Design review of the part shown in the three views and the two pictorial views. Dimensions are in mm from the part's minimum x, y and z. Round coordinates to 2 decimals unless told otherwise and drop trailing zeros. Loops run counter-clockwise (first coordinate to the right, second up) from the corner with the lowest first, then second, coordinate; pieces in that order, holes last. Notation, with made-up numbers: M 13,-2.75 L 18,-2.75 A32 ccw 18,24.25 Z; hole C 21.25,73.5 d10. An arc over 180 degrees is marked long. Return JSON: item names as keys, results as strings. Group by question number.
Q1. Consider section A-A (x = 7.5). State the section outline as (y, z) points.
Q2. To check wall thickness, follow line 1 along Z through (x, y) = (42.5, 3); line 2 along X through (y, z) = (1.65, 14); line 3 along X through (y, z) = (0.7, 22). State the ranges of each line that lie inside material, in increasing order.
Q3. Consider section B-B (z = 15). State the section outline as (x, y) points, and give its area (3 significant figures).
Q4. Clearance check with a flat-ended pin moving along its axis: pin 1 Ø4.5 at (x, z) = (24.5, 12) entering from -Y. State where the tip first meets the part, or that it passes through.
Q5. Consider section C-C (x = 24). State the section outline as (y, z) points, and give its area (3 significant figures).
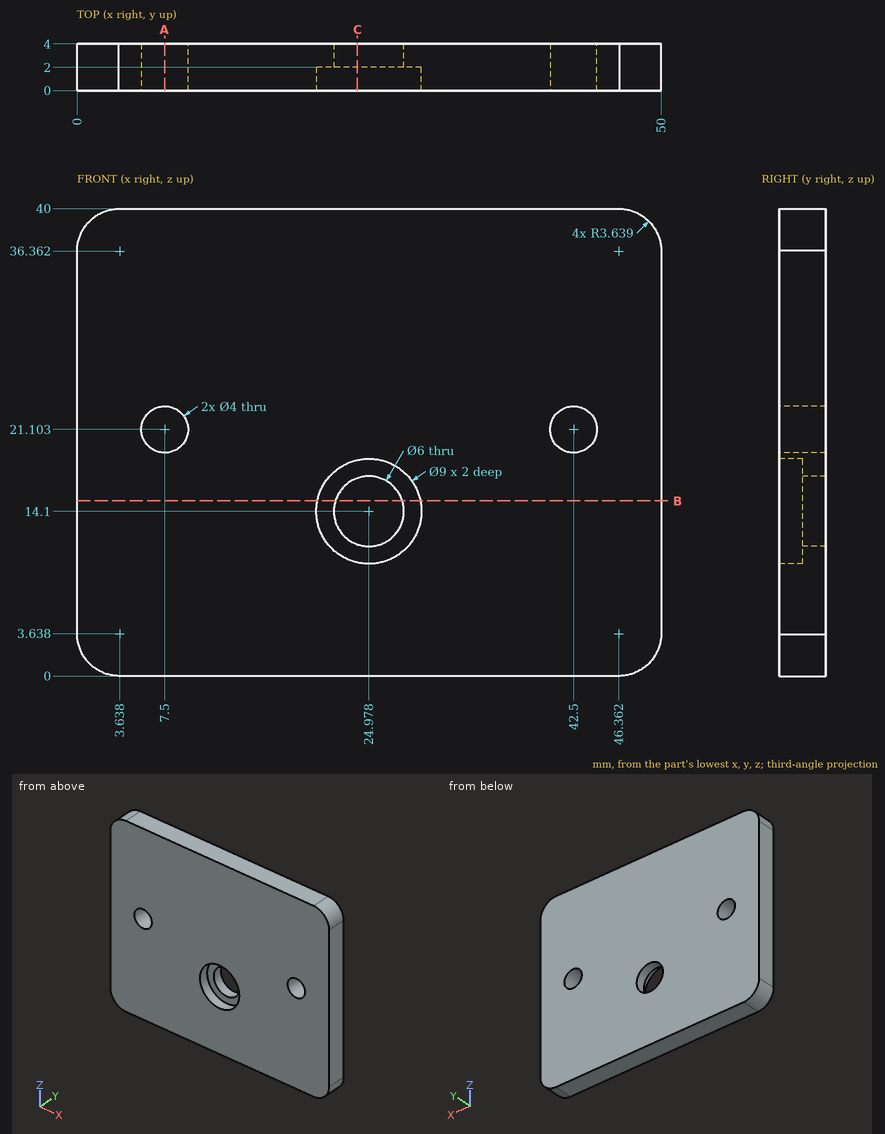
Values:
{
 "1": {"outline": "M 0,0 L 4,0 L 4,19.1 L 0,19.1 Z; M 0,23.1 L 4,23.1 L 4,40 L 0,40 Z"},
 "2": {"line 1": "z = 0 to 19.1, 23.1 to 40", "line 2": "x = 0 to 20.48, 29.48 to 50", "line 3": "x = 0 to 5.71, 9.29 to 40.71, 44.29 to 50"},
 "3": {"outline": "M 0,0 L 20.57,0 L 20.57,2 L 22.12,2 L 22.12,4 L 0,4 Z; M 27.84,2 L 29.39,2 L 29.39,0 L 50,0 L 50,4 L 27.84,4 Z", "area": "171 mm2"},
 "4": {"pin 1": "stops at y = 2"},
 "5": {"outline": "M 0,0 L 4,0 L 4,11.26 L 2,11.26 L 2,9.71 L 0,9.71 Z; M 0,18.49 L 2,18.49 L 2,16.94 L 4,16.94 L 4,40 L 0,40 Z", "area": "131 mm2"}
}
